```python
from build123d import *

# Parameters (mm, degrees)
F1_R      = 1
F2_DEPTH  = 6
F0_R      = 0.75
F3_DEPTH  = 9
F5_R      = 1.25
F6_DEPTH  = 3
F4_R      = 0.4
F7_DEPTH  = 2.36
F8_R      = 0.5
F9_DEPTH  = 2.63
F10_R     = 0.4
F11_DEPTH = 4.77


with BuildPart() as f2:
    # F1 (on Top) → F2 (new body)
    with BuildSketch(Plane.XY):
        Circle(F1_R)
    extrude(amount=F2_DEPTH)

    # F0 (on Top) → F3 (join)
    with BuildSketch(Plane.XY):
        Circle(F0_R)
    extrude(amount=F3_DEPTH)

    # F5 (on Top) → F6 (join)
    with BuildSketch(Plane.XY):
        Circle(F5_R)
    extrude(amount=F6_DEPTH)

    # F4 (on Top) → F7 (cut)
    with BuildSketch(Plane.XY):
        Circle(F4_R)
    extrude(amount=F7_DEPTH, mode=Mode.SUBTRACT)

    # F8 (on Top) → F9 (cut)
    with BuildSketch(Plane.XY):
        Circle(F8_R)
    extrude(amount=F9_DEPTH, mode=Mode.SUBTRACT)

    # F10 (on Top) → F11 (cut)
    with BuildSketch(Plane.XY):
        Circle(F10_R)
    extrude(amount=F11_DEPTH, mode=Mode.SUBTRACT)


solid = f2.part
```
Geometry check sheet. Reference: the model listing, model coordinates, mm. A direction names the side the tool comes from. Give positions to 0.01 mm unless a question says otherwise; leave off trailing zeros. Write each loop counter-clockwise with the first axis right and the second up, starting at its lowest first coordinate (ties: lowest second). Pieces come first, ordered by that corner, then holes. Notation, with made-up numbers: (41, -11.75) -> (73, -11.75) arc R9 cw to (73, -7.75) -> close; hole circle Ø9 at (1.5, 54). An arc over 180 degrees is marked (long way). One line per question, with ' | ' between items.
Item 1: Sectioned sample at C-C, the plane z = 0.5. Record the boundary of the cut face in (x, y), plus the area to 3 significant figures.
Determined:
outline: circle Ø2.5 at (0, 0); hole circle Ø1 at (0, 0) | area: 4.12 mm^2
Item 2: Sectioned sample at D-D, the plane z = 7.5. Record the boundary of the cut face in (x, y), plus the area to 3 significant figures.
Determined:
outline: circle Ø1.5 at (0, 0) | area: 1.77 mm^2
Item 3: Access from +Z, -Z, +X, -X, +Y, -Y to the whole of each face (thin tool, end or side, straight path). Record for faces 4 (the cylindrical face through (0, -1, 4)), 5 (the flat face through (0, -1, 0)).
Determined:
face 4: +Z | face 5: -Z, +X, -X, +Y, -Y
Item 4: Scan lines: line 1 along X through (y, z) = (0, 3.1); line 2 along Y through (x, z) = (0, 1.5). Record each from-to range of solid material in increasing order.
Determined:
line 1: -1 to -0.4, 0.4 to 1 | line 2: -1.25 to -0.5, 0.5 to 1.25
Item 5: Sectioned sample at A-A, the plane x = 0. Record the boundary of the cut face in (y, z).
Determined:
outline: (-1.25, 0) -> (-0.5, 0) -> (-0.5, 2.63) -> (-0.4, 2.63) -> (-0.4, 4.77) -> (0.4, 4.77) -> (0.4, 2.63) -> (0.5, 2.63) -> (0.5, 0) -> (1.25, 0) -> (1.25, 3) -> (1, 3) -> (1, 6) -> (0.75, 6) -> (0.75, 9) -> (-0.75, 9) -> (-0.75, 6) -> (-1, 6) -> (-1, 3) -> (-1.25, 3) -> close
Item 6: Depth check by flat-ended pin: pin 1 (1.5 mm diameter, centred on x = 1, z = 3, fed in from +Y); pin 2 (1.5 mm diameter, centred on x = 0.5, z = 5, fed in from +Y); pin 3 (1 mm diameter, centred on x = -0.5, z = 8, fed in from +Y). Enter the tip coordinate at first touch or a pass-through.
Determined:
pin 1: y = 1.22 | pin 2: y = 1 | pin 3: y = 0.75
Item 7: Draft check along X on faces 1 (the flat face through (0, 0, 9)), 2 (the cylindrical face through (-0.108, -0.488, 1.297)), 3 (the cylindrical face through (-0.75, 0.03, 7.48)). Enter one of: released by +X, released by -X, zero draft, split by the parting line, or undercut.
Determined:
face 1: zero draft | face 2: undercut | face 3: split by the parting line
